Design review of the part built by this model. Coordinates are the model's own, in mm. Face numbers are marked on the shaded views. Give positions to 0.01 mm unless a question says otherwise; leave off trailing zeros. Order: outer loops, then holes, each group sorted by start corner. A loop starts at its lowest first (then second) coordinate and runs counter-clockwise, first axis right, second up. Notation, with made-up numbers: M 86.25,82.5 L 105.25,82.5 A20 cw 105.25,105.5 Z; hole C -32,60 d1. An arc over 180 degrees is marked long. Answer as a JSON object with one key per item and string values.
from build123d import *

# Parameters (mm, degrees)
F0_R     = 9.525
F1_DEPTH = 30.6987799704
F1_TAPER = 3
F2_DEPTH = 50.8
F3_DEPTH = 44.45
F4_SIZE  = 5.08


with BuildPart() as f1:
    # F0 (on Front) → F1 (new body)
    with BuildSketch(Plane.XZ):
        with BuildLine():
            ThreePointArc((6.35, -37.5671066227), (29.099355663, -24.5934442484), (38.1, 0))
            ThreePointArc((38.1, 0), (29.099355663, 24.5934442484), (6.35, 37.5671066227))
            ThreePointArc((6.35, 37.5671066227), (-38.1, 0), (6.35, -37.5671066227))
        make_face()
        Circle(F0_R, mode=Mode.SUBTRACT)
    extrude(amount=F1_DEPTH, taper=F1_TAPER)

    # F0 (on Front) → F2 (join)
    with BuildSketch(Plane.XZ):
        with BuildLine():
            ThreePointArc((6.35, -37.5671066227), (29.099355663, -24.5934442484), (38.1, 0))
            ThreePointArc((38.1, 0), (29.099355663, 24.5934442484), (6.35, 37.5671066227))
            ThreePointArc((6.35, 37.5671066227), (-38.1, 0), (6.35, -37.5671066227))
        make_face()
        Circle(F0_R, mode=Mode.SUBTRACT)
    extrude(amount=F2_DEPTH)

    # F0 (on Front) → F3 (join)
    with BuildSketch(Plane.XZ):
        with BuildLine():
            ThreePointArc((6.35, 37.5671066227), (29.099355663, 24.5934442484), (38.1, 0))
            ThreePointArc((38.1, 0), (29.099355663, -24.5934442484), (6.35, -37.5671066227))
            Line((6.35, -37.5671066227), (80.4333333333, -25.0447377485))
            ThreePointArc((80.4333333333, -25.0447377485), (50.8, 0), (80.4333333333, 25.0447377485))
            Line((80.4333333333, 25.0447377485), (6.35, 37.5671066227))
        make_face()
        with BuildLine():
            ThreePointArc((101.6, 0), (95.599570442, 16.3956294989), (80.4333333333, 25.0447377485))
            ThreePointArc((80.4333333333, 25.0447377485), (50.8, 0), (80.4333333333, -25.0447377485))
            ThreePointArc((80.4333333333, -25.0447377485), (95.599570442, -16.3956294989), (101.6, 0))
        make_face()
        with Locations((76.2, 0)):
            Circle(F0_R, mode=Mode.SUBTRACT)
    extrude(amount=F3_DEPTH)

    # F4
    f4_edges = [f1.edges().sort_by_distance(p)[0] for p in [
        (-9.525, -50.8, 0),
        (-6.35, -50.8, 37.567107),
        (66.675, -44.45, 0),
    ]]
    chamfer(f4_edges, length=F4_SIZE)


solid = f1.part
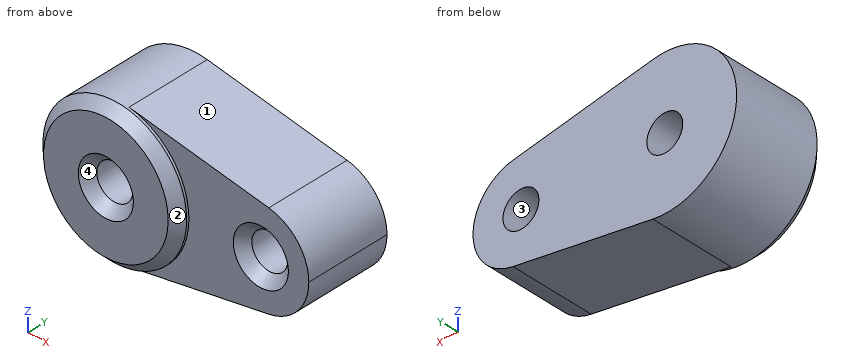
(1) To check wall thickness, follow L1, parallel to X at y = -2.5, z = -1.5; L2, parallel to Y at x = 34.5, z = 31; L3, parallel to Z at x = 3, y = -16.5. State the ranges of each line that lie inside material, in increasing order. Write a range as from..to.
Checked values:
{"L1": "x = -38.07..-9.41, 9.41..66.79, 85.61..101.56", "L2": "y = -44.45..0", "L3": "z = -37.98..-9.04, 9.04..37.98"}
(2) We need section D-D (z = -2.5). Count the separate pieces of the cut face and the enclosed holes in it, plus the area to 3 significant figures.
Checked values:
{"separate pieces": "3", "enclosed holes": "0", "area": "4,850 mm^2"}
(3) We need section C-C (x = 76.2). Write out the cut boundary in (y, z) (3 decimals).
Checked values:
{"outline": "M -44.45,-25.76 L 0,-25.76 L 0,-9.525 L -39.37,-9.525 L -44.45,-14.605 Z; M -44.45,14.605 L -39.37,9.525 L 0,9.525 L 0,25.76 L -44.45,25.76 Z"}
(4) Insertion check: pin 1 (8 mm diameter, centred on y = -25.5, z = -5.5, fed in from +X); pin 2 (4 mm diameter, centred on x = 61, y = -33.5, fed in from -Z); pin 3 (1 mm diameter, centred on y = -15.5, z = 23, fed in from +X). Each pin has a flat end and moves straight along its axis. Give the tip position at first contact, or say it passes through.
Checked values:
{"pin 1": "stops at x = 101.56", "pin 2": "stops at z = -28.67", "pin 3": "stops at x = 87.99"}
(5) We need section B-B (y = -13). Write out the cut boundary in (x, z) (3 decimals).
Checked values:
{"outline": "M 6.35,-37.567 L 80.433,-25.045 A25.4 ccw 80.433,25.045 L 6.35,37.567 A38.1 ccw long Z; hole C 0,0 d19.05; hole C 76.2,0 d19.05"}
(6) Draft analysis for pull direction Z (two halves, no side actions). For the marked faces 1, 2, 3 and 4, state which applies: +Z half, -Z half, draft (parallel to the pull), parting line (faces both ways), or undercut.
Checked values:
{"face 1": "+Z half", "face 2": "parting line", "face 3": "undercut", "face 4": "undercut"}
(7) We need section A-A (x = 0). Write out the cut boundary in (y, z) (3 decimals).
Checked values:
{"outline": "M -50.8,-33.02 L -45.72,-38.1 L 0,-38.1 L 0,-9.525 L -45.72,-9.525 L -50.8,-14.605 Z; M -50.8,14.605 L -45.72,9.525 L 0,9.525 L 0,38.1 L -45.72,38.1 L -50.8,33.02 Z"}
